The listing builds one solid part. Answer for the finished solid, in the listing's coordinates (mm). Face numbers are marked on the shaded views. A direction names the side the tool comes from. Coordinates: 2 decimals unless noted, no trailing zeros. Order: outer loops, then holes, each group sorted by start corner. A loop starts at its lowest first (then second) coordinate and runs counter-clockwise, first axis right, second up. Notation, with made-up numbers: (86, -13) - (129, -13) arc R16 cw to (129, 18) - close; hole circle Ø2 at (46.25, 82.5). An arc over 180 degrees is marked (long way). Use one line per item in the form item = value. Start each with the question number.
Item 1: Each of these flat-tipped pins is pushed along its axis until it touches: pin 1 Ø3 at (y, z) = (-220.5, 5) entering from +X (3 decimals); pin 2 Ø5.5 at (x, y) = (-11.11, -219.08) entering from -Z (3 decimals). Where does it stop, or does it pass through?
Item 2: The mould has two halves that part along Z. Classify the marked faces 3, 4 and 5: released by +Z, released by -Z, zero draft, split by the parting line, or undercut.
Item 3: Section A-A, the plane x = -5 is taken. Write down the section's boundary in (y, z) (3 decimals).
Item 4: Section B-B, the plane y = -92.5 is taken. Write down the section's boundary in (x, z) (3 decimals).
Item 5: A tool of negligible diameter and unlimited length cuts with its end or side. For the marked faces 1 and 2, from which of +Z, -Z, +X, -X, +Y, -Y can it reach the whole face along a straight path? Write none if from no direction.
Item 6: Section C-C, the plane z = -5.5 is taken. Write down the section's boundary in (x, y) (3 decimals), and give its area (3 significant figures).
Item 7: Consider line 1 along Z through (x, y) = (-15.25, -32) (3 decimals); line 2 along X through (y, z) = (-59.5, -11.5) (3 decimals). Determine where each line is inside the solid, lowest interval first. Write a range as [from, to].
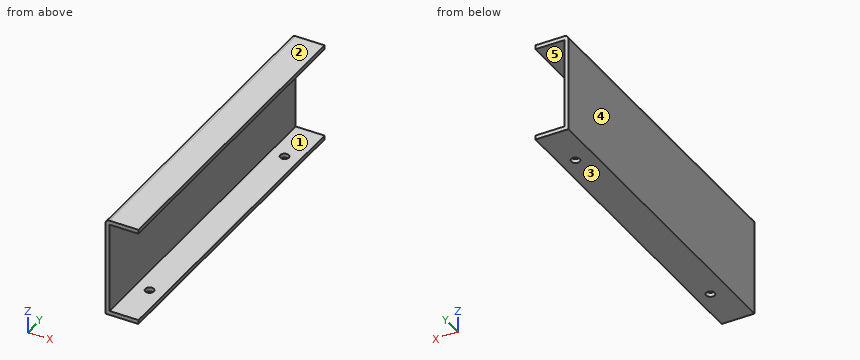
from build123d import *

# Parameters (mm, degrees)
F1_DEPTH = 254
F3_D     = 6.6
F3_DEPTH = 15
F3_TIP   = 1.9828400428
F4_R     = 3.175


with BuildPart() as f1:
    # F0 (on Front) → F1 (new body)
    with BuildSketch(Plane.XZ):
        Polygon((0, 34.925), (0, 38.1), (-25.4, 38.1), (-25.4, -38.1), (0, -38.1), (0, -34.925), (-22.225, -34.925), (-22.225, 34.925), align=None)
    extrude(amount=F1_DEPTH)

    # F3
    with Locations(Plane(origin=(0, 0, -38.1), x_dir=(1, 0, 0), z_dir=(0, 0, -1))):
        with Locations((-11.1125, 219.075), (-11.1125, 34.925)):
            Hole(F3_D / 2, depth=F3_DEPTH)
            with Locations((0, 0, -(F3_DEPTH + F3_TIP / 2))):  # 118° drill point
                Cone(0, F3_D / 2, F3_TIP, mode=Mode.SUBTRACT)

    # F4
    f4_edges = [f1.edges().sort_by_distance(p)[0] for p in [
        (-25.4, -127, 38.1),
    ]]
    fillet(f4_edges, radius=F4_R)


solid = f1.part
Response:
q1.pin_1 = -22.225
q1.pin_2 = 34.925
q2.face_3 = released by -Z
q2.face_4 = zero draft
q2.face_5 = undercut
q3.outline = (-254, -38.1) - (0, -38.1) - (0, -34.925) - (-254, -34.925) - close; (-254, 34.925) - (0, 34.925) - (0, 38.1) - (-254, 38.1) - close
q4.outline = (-25.4, -38.1) - (0, -38.1) - (0, -34.925) - (-22.225, -34.925) - (-22.225, 34.925) - (0, 34.925) - (0, 38.1) - (-22.225, 38.1) arc R3.175 ccw to (-25.4, 34.925) - close
q5.face_1 = +X, +Y, -Y
q5.face_2 = +Z, +X, -X, +Y, -Y
q6.outline = (-25.4, -254) - (-22.225, -254) - (-22.225, 0) - (-25.4, 0) - close
q6.area = 806 mm2
q7.line_1 = [-38.1, -34.925], [34.925, 38.1]
q7.line_2 = [-25.4, -22.225]
